Design review of the part built by this model. Coordinates are the model's own, in mm. A direction names the side the tool comes from. Give positions to 0.01 mm unless a question says otherwise; leave off trailing zeros. Loops run counter-clockwise (first coordinate to the right, second up) from the corner with the lowest first, then second, coordinate; pieces in that order, holes last. Notation, with made-up numbers: M 80,42.25 L 94,42.25 A11 cw 94,60.25 Z; hole C 88.25,46.5 d7. An arc over 180 degrees is marked long. Answer as CSV lines item,"result".
```python
from build123d import *

# Parameters (mm, degrees)
SKETCH1_W           = 135
SKETCH1_H           = 56
BOSS_EXTRUDE1_DEPTH = 28
SKETCH2_R           = 36
BOSS_EXTRUDE2_DEPTH = 55
SKETCH3_W           = 18
SKETCH3_H           = 32
CUT_EXTRUDE1_DEPTH  = 20
CUT_EXTRUDE2_START  = -24
CUT_EXTRUDE2_DEPTH  = 24


with BuildPart() as part:
    # Sketch1 → Boss-Extrude1 (new body)
    with BuildSketch(Plane(origin=(0, 0, 0), x_dir=(1, 0, 0), z_dir=(0, 1, 0))):
        Rectangle(SKETCH1_W, SKETCH1_H)
    extrude(amount=BOSS_EXTRUDE1_DEPTH)

    # Sketch2 → Boss-Extrude2 (add)
    with BuildSketch(Plane(origin=(0, 0, 0), x_dir=(1, 0, 0), z_dir=(0, 1, 0))):
        with Locations(Location((0, 0, 0), (0, 0, 51.057558731))):
            Circle(SKETCH2_R)
    extrude(amount=BOSS_EXTRUDE2_DEPTH)

    # Sketch3 → Cut-Extrude1 (cut)
    with BuildSketch(Plane(origin=(0, 28, 0), x_dir=(1, 0, 0), z_dir=(0, 1, 0))):
        with Locations((-58.5, 0)):
            Rectangle(SKETCH3_W, SKETCH3_H)
    cut_extrude1 = extrude(amount=-CUT_EXTRUDE1_DEPTH, mode=Mode.SUBTRACT)

    # Mirror1: Cut-Extrude1 across plane
    add(cut_extrude1.mirror(Plane(origin=(0, 0, 0), x_dir=(0, 0, 1), z_dir=(1, 0, 0))), mode=Mode.SUBTRACT)

    # Sketch4 → Cut-Extrude2 (cut)
    with BuildSketch(Plane(origin=(0, 55, 0), x_dir=(1, 0, 0), z_dir=(0, 1, 0)).offset(CUT_EXTRUDE2_START)):
        with BuildLine():
            Line((-13, 33.570820663), (-13, 21.354156504))
            ThreePointArc((-13, 21.354156504), (-25, 0), (-13, -21.354156504))
            Line((-13, -21.354156504), (-13, -33.570820663))
            ThreePointArc((-13, -33.570820663), (0, -36), (13, -33.570820663))
            Line((13, -33.570820663), (13, -21.354156504))
            ThreePointArc((13, -21.354156504), (25, 0), (13, 21.354156504))
            Line((13, 21.354156504), (13, 33.570820663))
            ThreePointArc((13, 33.570820663), (0, 36), (-13, 33.570820663))
        make_face()
    extrude(amount=CUT_EXTRUDE2_DEPTH, mode=Mode.SUBTRACT)


solid = part.part
```
1. We need section C-C, the plane y = 3. Write out the cut boundary in (x, z), plus the area to 3 significant figures.
Answer block:
outline,"M -67.5,-28 L -22.63,-28 A36 ccw 22.63,-28 L 67.5,-28 L 67.5,28 L 22.63,28 A36 ccw -22.63,28 L -67.5,28 Z"
area,"8,050 mm²"
2. The part is to be moulded in two halves that separate along X. For faces 4 (the flat face through (-45, 14, 28)), 5 (the flat face through (-67.5, 7.6, 0.4)), 6 (the flat face through (0, 31, -1)), say which applies: pulls with the +X half, pulls with the -X half, needs draft (parallel to the pull), parting line crosses it, or undercut.
Answer block:
face 4,"needs draft"
face 5,"pulls with the -X half"
face 6,"undercut"
3. We need section B-B, the plane z = 0. Write out the cut boundary in (x, y), plus the area to 3 significant figures.
Answer block:
outline,"M -67.5,0 L 67.5,0 L 67.5,8 L 49.5,8 L 49.5,28 L 36,28 L 36,55 L 25,55 L 25,31 L -25,31 L -25,55 L -36,55 L -36,28 L -49.5,28 L -49.5,8 L -67.5,8 Z"
area,"3,800 mm²"
4. For faces 1 (the flat face through (-13, 43, 27)), 2 (the flat face through (45, 14, 28)), 3 (the flat face through (-59, 18, 16)), list the 3-axis set-ups (+Z, -Z, +X, -X, +Y, -Y) from which the entire face can be reached by the end or side of a thin tool; tool diameter is ignored.
Answer block:
face 1,"+Z, -Z, +Y"
face 2,"+Z, +X, +Y, -Y"
face 3,"-X, +Y"
5. To check wall thickness, follow L1, parallel to X at y = 48.5, z = 29; L2, parallel to Z at x = 53, y = 19.5; L3, parallel to X at y = 14.5, z = -5.5. State the ranges of each line that lie inside material, in increasing order. Write a range as [from, to].
Answer block:
L1,"[-21.33, -13], [13, 21.33]"
L2,"[-28, -16], [16, 28]"
L3,"[-49.5, 49.5]"
6. For P1, Ø14, axis at x = -53.5, y = 19, coming from the +Z side; P2, Ø6, axis at x = -17.5, y = 31, coming from the -Z side; P3, Ø5, axis at y = 13.5, z = 7, coming from the +X side, all flat-tipped, find the tip position at first contact; note any pin that passes through.
Answer block:
P1,"z = 28"
P2,"z = -32.95"
P3,"x = 49.5"
7. We need section D-D, the plane x = -19. Write out the cut boundary in (y, z).
Answer block:
outline,"M 0,-30.58 L 55,-30.58 L 55,-16.25 L 31,-16.25 L 31,16.25 L 55,16.25 L 55,30.58 L 0,30.58 Z"
8. We need section A-A, the plane y = 51. Write out the cut boundary in (x, z).
Answer block:
outline,"M -13,-33.57 L -13,-21.35 A25 cw -13,21.35 L -13,33.57 A36 ccw Z; M 13,-33.57 A36 ccw 13,33.57 L 13,21.35 A25 cw 13,-21.35 Z"
